Verification items for the finished model (mm, model axes). A direction names the side the tool comes from. Give positions to 0.01 mm unless a question says otherwise; leave off trailing zeros. Loops run counter-clockwise (first coordinate to the right, second up) from the corner with the lowest first, then second, coordinate; pieces in that order, holes last. Notation, with made-up numbers: (-2.5, 60.25) -> (53.5, 60.25) arc R11 ccw to (53.5, 69.25) -> close; hole circle Ø11 at (57.5, 53). An arc over 180 degrees is marked (long way). Answer in a Markdown table with one row per item. Add a question column.
Q1. Section check A-A on y = 13. Enter the section's corners in (x, z), and give its area (3 significant figures).
Q2. Gauge pin test, flat ends, axial feed: P1, Ø2, axis at x = 59, z = -54, coming from the +Y side; P2, Ø7.5, axis at y = -4, z = -17.5, coming from the -X side; P3, Ø20, axis at x = 74, z = -45, coming from the -Y side. Record the tip position at first contact, or that the pin passes through.
Q3. Release check for a two-part mould opening along Z. For faces 1 (the face through (34, 11, 0)), 2 (the face through (74, 0, -32)), 3 (the face through (52.94, 7.2, -26.91)) record: pulls with the +Z half, pulls with the -Z half, needs draft (parallel to the pull), parting line crosses it, or undercut.
Q4. Section check C-C on y = 23. Enter the section's corners in (x, z), and give its area (3 significant figures).
Q5. Section check B-B on x = 50. Enter the section's corners in (y, z), and give its area (3 significant figures).
Q6. Set-up check for faces 4 (the face through (16, 0, -32)), 5 (the face through (61, -3, -32)), 6 (the face through (54, 26, -58)), 7 (the face through (56, 21, -32)): record each of +Z, -Z, +X, -X, +Y, -Y from which the full face is reachable in a straight line by a thin tool's end or side.
Q7. Section check D-D on z = -6. Enter the section's corners in (x, y), and give its area (3 significant figures).
Q8. Material ranges on probe 1 along X at (y, z) = (15, -26); probe 2 along Y at (x, z) = (45, -35.5); probe 3 along Y at (x, z) = (10.5, -16), recorded low to high.
```python
from build123d import *

# Parameters (mm, degrees)
BOSS_EXTRUDE1_DEPTH = 64
CUT_EXTRUDE1_DEPTH  = 93.374238833
SKETCH4_R           = 7
CUT_EXTRUDE2_DEPTH  = 18
CUT_EXTRUDE7_REACH  = 118.653
SKETCH4_6_R         = 7
CUT_EXTRUDE8_START  = -18
CUT_EXTRUDE8_DEPTH  = 9


with BuildPart() as part:
    # Sketch1 → Boss-Extrude1 (new body)
    with BuildSketch(Plane.XY):
        Polygon((0, 0), (0, 39), (54, 39), (54, 21), (86, 21), (86, 0), (61, 0), (61, -7), (31, -7), (31, 0), align=None)
    extrude(amount=-BOSS_EXTRUDE1_DEPTH)

    # Sketch3 → Cut-Extrude1 (cut, through all)
    with BuildSketch(Plane(origin=(54, 0, 0), x_dir=(0, 0, -1), z_dir=(1, 0, 0))):
        Polygon((40, 39), (64, 27.808616204), (64, 39), align=None)
    extrude(amount=-CUT_EXTRUDE1_DEPTH, mode=Mode.SUBTRACT)

    # Sketch4 → Cut-Extrude2 (cut)
    # profile 1 of 2: a face of its own
    with BuildSketch(Plane(origin=(0, 39, 0), x_dir=(1, 0, 0), z_dir=(0, 1, 0))):
        Polygon((54, 40), (54, 52), (43.930804426, 40), align=None)
    # profile 2 of 2: a face of its own
    with BuildSketch(Plane(origin=(0, 39, 0), x_dir=(1, 0, 0), z_dir=(0, 1, 0))):
        Polygon((54, 40), (43.930804426, 40), (10.366819179, 0), (54, 0), align=None)
        with Locations(Location((46, 26, 0), (0, 0, 270))):
            Circle(SKETCH4_R, mode=Mode.SUBTRACT)
    extrude(amount=-CUT_EXTRUDE2_DEPTH, mode=Mode.SUBTRACT)

    # Sketch4_6 → Cut-Extrude7 (cut, up to next)
    with BuildSketch(Plane(origin=(0, 39, 0), x_dir=(1, 0, 0), z_dir=(0, 1, 0)), mode=Mode.PRIVATE) as cut_extrude7_sk1:
        with Locations(Location((46, 26, 0), (0, 0, 270))):
            Circle(SKETCH4_6_R)
    cut_extrude7_tool1 = extrude(cut_extrude7_sk1.sketch, amount=-CUT_EXTRUDE7_REACH, mode=Mode.PRIVATE) & part.part
    add(cut_extrude7_tool1.solids().sort_by_distance((46, 39, -26))[0], mode=Mode.SUBTRACT)

    # Sketch4_7 → Cut-Extrude8 (cut)
    with BuildSketch(Plane(origin=(0, 39, 0), x_dir=(1, 0, 0), z_dir=(0, 1, 0)).offset(CUT_EXTRUDE8_START)):
        Polygon((86, 26), (86, -0.057865332), (61, -0.057865332), align=None)
    extrude(amount=-CUT_EXTRUDE8_DEPTH, mode=Mode.SUBTRACT)


solid = part.part
```
Taken from the geometry:
| question | item | result |
|---|---|---|
| 1 | outline | (0, -64) -> (86, -64) -> (86, -26) -> (61.06, 0) -> (0, 0) -> close; hole circle Ø14 at (46, -26) |
| 1 | area | 5,030 mm² |
| 2 | P1 | stops at y = 21 |
| 2 | P2 | stops at x = 31 |
| 2 | P3 | stops at y = 0 |
| 3 | face 1 | pulls with the +Z half |
| 3 | face 2 | needs draft |
| 3 | face 3 | undercut |
| 4 | outline | (0, -64) -> (54, -64) -> (54, -52) -> (10.37, 0) -> (0, 0) -> close |
| 4 | area | 2,320 mm² |
| 5 | outline | (-7, -64) -> (27.81, -64) -> (35.63, -47.23) -> (21, -47.23) -> (21, -31.74) -> (-7, -31.74) -> close; (-7, -20.26) -> (21, -20.26) -> (21, 0) -> (-7, 0) -> close |
| 5 | area | 1,650 mm² |
| 6 | face 4 | +Z, -Z, -X, -Y |
| 6 | face 5 | +Z, -Z, +X, -Y |
| 6 | face 6 | +Z, -Z, +X, +Y |
| 6 | face 7 | +Z, +X, +Y |
| 7 | outline | (0, 0) -> (31, 0) -> (31, -7) -> (61, -7) -> (61, 0) -> (86, 0) -> (86, 12) -> (66.81, 12) -> (66.81, 21) -> (15.4, 21) -> (15.4, 39) -> (0, 39) -> close |
| 7 | area | 2,120 mm² |
| 8 | probe 1 | x = 0 to 39, 53 to 86 |
| 8 | probe 2 | y = -7 to 21 |
| 8 | probe 3 | y = 0 to 39 |
